Verification items for the finished model (mm, model axes). Face numbers are marked on the shaded views. A direction names the side the tool comes from. Coordinates: 2 decimals unless noted, no trailing zeros. Write each loop counter-clockwise with the first axis right and the second up, starting at its lowest first coordinate (ties: lowest second). Pieces come first, ordered by that corner, then holes. Notation, with made-up numbers: (31.5, 1.25) -> (49.5, 1.25) arc R23 cw to (49.5, 12.25) -> close; hole circle Ø3 at (63.25, 84.5). An arc over 180 degrees is marked (long way). Write item = value, one per line. Start each with the question number.
(1) Gauge pin test, flat ends, axial feed: pin 1 Ø3.5 at (y, z) = (5, -7) entering from +X; pin 2 Ø5.5 at (x, z) = (29, -14) entering from +Y; pin 3 Ø5 at (x, z) = (-10, 0) entering from +Y; pin 4 Ø2.5 at (x, z) = (0, -15) entering from -Y. Record the tip position at first contact, or that the pin passes through.
(2) Section check A-A (x = 37). Record the cut outline in (y, z).
(3) Set-up check for the marked faces 1, 2 and 3: record each of +Z, -Z, +X, -X, +Y, -Y from which the full face is reachable in a straight line by a thin tool's end or side.
(4) Section check B-B (x = 0). Record the cut outline in (y, z).
(5) Section check D-D (z = -0.5). State how many separate pieces and enclosed holes the cut face has, plus the area to 3 significant figures.
(6) Material ranges on probe 1 along X at (y, z) = (1.05, 0); probe 2 along X at (y, z) = (5.35, 0); probe 3 along X at (y, z) = (2.85, 14), recorded low to high. Write a range as [from, to].
(7) Mould release check, pull along X, two halves, no side actions. Record for the marked faces 4, 5, 6 and 7: released by +X, released by -X, zero draft, split by the parting line, or undercut.
(8) Section check C-C (z = -7). Record the cut outline in (x, y).
```python
from build123d import *

# Parameters (mm, degrees)
SKETCH_1_R          = 1.5
EXTRUDE_1_DEPTH     = 6
SKETCH_2_W          = 7
SKETCH_2_H          = 5
CUT_EXTRUDE_1_DEPTH = 3
SKETCH_3_R          = 3.5
CUT_EXTRUDE_2_DEPTH = 1.5
SKETCH_5_R          = 3
CUT_EXTRUDE_3_DEPTH = 3
SKETCH_6_R          = 6
EXTRUDE_2_DEPTH     = 3.5
CUT_EXTRUDE_START   = -1
SKETCH_7_R          = 3
CUT_EXTRUDE_4_DEPTH = 1
SKETCH_8_R          = 1.5
CUT_EXTRUDE_5_DEPTH = 49.179352424
FILLET_1_R          = 1


with BuildPart() as part:
    # 草图1 → 凸台-拉伸1 (new body)
    with BuildSketch(Plane(origin=(0, 0, 0), x_dir=(1, 0, 0), z_dir=(0, 1, 0))):
        Polygon((-27, 15), (-27, -15), (-5, -15), (-5, -20), (5, -20), (5, -15), (22, -15), (27, -20), (35, -20), (35, -12), (43, -4), (43, 4), (35, 12), (35, 20), (27, 20), (22, 15), (5, 15), (5, 20), (-5, 20), (-5, 15), align=None)
        with Locations(Location((0, 15, 0), (0, 0, 270))):
            Circle(SKETCH_1_R, mode=Mode.SUBTRACT)
        with Locations(Location((0, -15, 0), (0, 0, 270))):
            Circle(SKETCH_1_R, mode=Mode.SUBTRACT)
        with Locations(Location((29, 14, 0), (0, 0, 270))):
            Circle(SKETCH_1_R, mode=Mode.SUBTRACT)
        with Locations(Location((37, 0, 0), (0, 0, 270))):
            Circle(SKETCH_1_R, mode=Mode.SUBTRACT)
        with Locations(Location((29, -14, 0), (0, 0, 270))):
            Circle(SKETCH_1_R, mode=Mode.SUBTRACT)
    extrude(amount=EXTRUDE_1_DEPTH)

    # 草图2 → 切除-拉伸1 (cut)
    with BuildSketch(Plane(origin=(0, 6, 0), x_dir=(1, 0, 0), z_dir=(0, 1, 0))):
        with Locations((-23.5, 2.5)):
            Rectangle(SKETCH_2_W, SKETCH_2_H)
        with Locations((-23.5, -2.5)):
            Rectangle(SKETCH_2_W, SKETCH_2_H)
        Polygon((20, 10), (-20, 10), (-20, 5), (-20, 0), (20, 0), align=None)
        Polygon((20, 0), (-20, 0), (-20, -5), (-20, -10), (20, -10), align=None)
    extrude(amount=-CUT_EXTRUDE_1_DEPTH, mode=Mode.SUBTRACT)

    # 草图3 → 切除-拉伸2 (cut)
    with BuildSketch(Plane(origin=(0, 6, 0), x_dir=(1, 0, 0), z_dir=(0, 1, 0))):
        with Locations(Location((0, 15, 0), (0, 0, 270))):
            Circle(SKETCH_3_R)
        with Locations(Location((0, -15, 0), (0, 0, 270))):
            Circle(SKETCH_3_R)
        with Locations(Location((29, -14, 0), (0, 0, 270))):
            Circle(SKETCH_3_R)
        with Locations(Location((37, 0, 0), (0, 0, 270))):
            Circle(SKETCH_3_R)
        with Locations(Location((29, 14, 0), (0, 0, 270))):
            Circle(SKETCH_3_R)
    extrude(amount=-CUT_EXTRUDE_2_DEPTH, mode=Mode.SUBTRACT)

    # 草图5 → 切除-拉伸3 (cut)
    with BuildSketch(Plane(origin=(0, 3, 0), x_dir=(1, 0, 0), z_dir=(0, 1, 0))):
        with Locations(Location((-10, 0, 0), (0, 0, 270))):
            Circle(SKETCH_5_R)
    extrude(amount=-CUT_EXTRUDE_3_DEPTH, mode=Mode.SUBTRACT)

    # 草图6 → 凸台-拉伸2 (add)
    with BuildSketch(Plane.XZ):
        with Locations(Location((-10, 0, 0), (0, 0, 90))):
            Circle(SKETCH_6_R)
    extrude(amount=EXTRUDE_2_DEPTH)

    # 草图7 → 切除-拉伸4 (cut)
    with BuildSketch(Plane.XZ.offset(3.5).offset(CUT_EXTRUDE_START)):
        with Locations(Location((-10, 0, 0), (0, 0, 90))):
            Circle(SKETCH_7_R)
    extrude(amount=CUT_EXTRUDE_4_DEPTH, mode=Mode.SUBTRACT)

    # 草图8 → 切除-拉伸5 (cut, through all)
    with BuildSketch(Plane.XZ.offset(2.5)):
        with Locations(Location((-10, 0, 0), (0, 0, 270))):
            Circle(SKETCH_8_R)
    extrude(amount=-CUT_EXTRUDE_5_DEPTH, mode=Mode.SUBTRACT)

    # 圆角1
    fillet_1_edges = [part.edges().sort_by_distance(p)[0] for p in [
        (22, 3, -15),
        (22, 3, 15),
        (5, 3, 15),
        (5, 3, 20),
        (-5, 3, 20),
        (-5, 3, 15),
        (-27, 3, 15),
        (-27, 3, -15),
        (-5, 3, -15),
        (-5, 3, -20),
        (5, 3, -20),
        (5, 3, -15),
    ]]
    fillet(fillet_1_edges, radius=FILLET_1_R)


solid = part.part
```
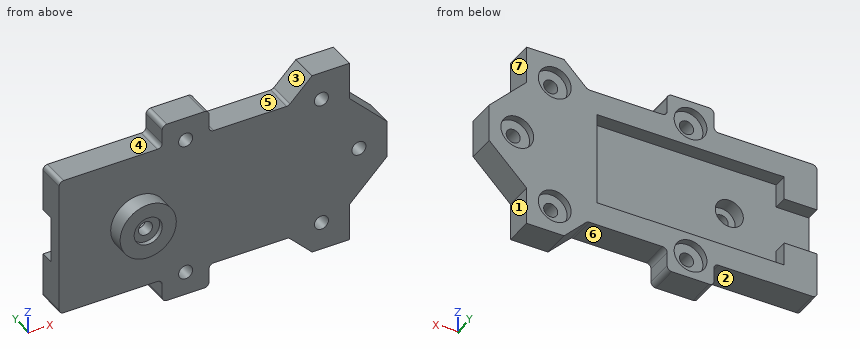
Response:
q1.pin_1 = 41.75
q1.pin_2 = 4.5
q1.pin_3 = 0
q1.pin_4 = through
q2.outline = (0, -10) -> (6, -10) -> (6, -3.5) -> (4.5, -3.5) -> (4.5, -1.5) -> (0, -1.5) -> close; (0, 1.5) -> (4.5, 1.5) -> (4.5, 3.5) -> (6, 3.5) -> (6, 10) -> (0, 10) -> close
q3.face_1 = -Z, +X, +Y, -Y
q3.face_2 = -Z, -X, +Y, -Y
q3.face_3 = +Z, +Y, -Y
q4.outline = (0, -20) -> (6, -20) -> (6, -18.5) -> (4.5, -18.5) -> (4.5, -16.5) -> (0, -16.5) -> close; (0, -13.5) -> (4.5, -13.5) -> (4.5, -11.5) -> (6, -11.5) -> (6, -10) -> (3, -10) -> (3, 10) -> (6, 10) -> (6, 11.5) -> (4.5, 11.5) -> (4.5, 13.5) -> (0, 13.5) -> close; (0, 16.5) -> (4.5, 16.5) -> (4.5, 18.5) -> (6, 18.5) -> (6, 20) -> (0, 20) -> close
q5.separate_pieces = 3
q5.enclosed_holes = 0
q5.area = 267 mm2
q6.probe_1 = [-27, -13], [-7, 35.5], [38.5, 43]
q6.probe_2 = [20, 33.5], [40.5, 43]
q6.probe_3 = [-27, -1.12], [1.12, 27.5], [30.5, 35]
q7.face_4 = zero draft
q7.face_5 = undercut
q7.face_6 = undercut
q7.face_7 = released by +X
q8.outline = (-27, 0) -> (40, 0) -> (40, 6) -> (20, 6) -> (20, 3) -> (-20, 3) -> (-20, 6) -> (-27, 6) -> close
